Read the model definition and answer for the solid it produces. Units are mm, in the model's axes. Round coordinates to 2 decimals unless told otherwise and drop trailing zeros. Order: outer loops, then holes, each group sorted by start corner. A loop starts at its lowest first (then second) coordinate and runs counter-clockwise, first axis right, second up. Notation, with made-up numbers: (7, 72) - (40, 72) arc R29 cw to (40, 95) - close; hole circle Ø11 at (49.25, -22). An arc over 180 degrees is marked (long way). Put each result on its own line as item: value. Start each with the question number.
Q1. Section D-D on z = -3.75 is taken. Give the vertices of the cut face in (x, y).
Q2. Section B-B on x = -74 is taken. Give the vertices of the cut face in (y, z) (3 decimals), then the cut area to 3 significant figures.
Q3. Find the intervals of material crossed by line 1 along X through (y, z) = (0.75, -10.3); line 2 along X through (y, z) = (1.6, -11.75); line 3 along Y through (x, z) = (-8, -5), in increasing order. Write a range as from..to.
Q4. Section C-C on y = 1.35 is taken. Give the vertices of the cut face in (x, z).
Q5. This flat-tipped pin is pushed along its axis until it touches: pin 1 Ø1 at (x, z) = (-90, -5) entering from -Y. Where does it stop, or does it pass through?
Q6. Section A-A on z = -10.3 is taken. Give the vertices of the cut face in (x, y), then the cut area to 3 significant figures.
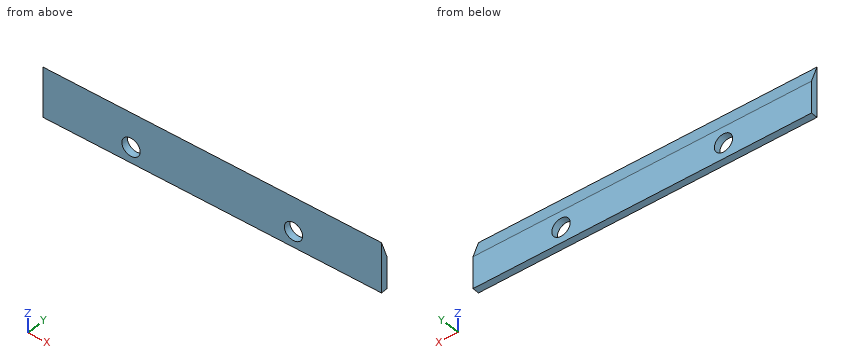
Autodesk Inventor part; units mm, degrees
ref_plane "Work Plane1" through (-50, 0, -15) normal (1, 0, 0) x (0, 0, -1)
ref_plane "YZ Plane" through (0, 0, 0) normal (1, 0, 0) x (0, 1, 0)
ref_plane "XZ Plane" through (0, 0, 0) normal (0, 1, 0) x (-1, 0, 0)
sketch "Sketch1" plane through (0, 0, 0) normal (0, 1, 0) x (-1, 0, 0)
  line L0 (0, 0) -> (100, 0)
  line L1 (100, 0) -> (100, -15)
  line L2 (100, -15) -> (0, -15)
  line L3 (0, -15) -> (0, 0)
  dimension "d0" = 100
  dimension "d1" = 15
extrude "Extrusion1" add sketch "Sketch1" along normal blind 2
sketch "Sketch2" plane through (0, 0, 0) normal (1, 0, 0) x (0, 0, -1)
  line L0 (0, 0) -> (0, 2)
  line L1 (0, 0) -> (5.495, 2)
  line L2 (5.495, 2) -> (5.495, 0)
  line L3 (5.495, 0) -> (0, 0)
  line L4 (0, 2) -> (15, 2)
  dimension "d4" = 20
extrude "Extrusion2" cut sketch "Sketch2" against normal through all contours L0 L4 L1
sketch "Sketch3" plane through (0, 2, 0) normal (0, 1, 0) x (1, 0, 0)
  line L0 (-100, 15) -> (-100, 5.495)
  point P0 (0, 0)
  point P1 (-74, 10.3)
  point P2 (-100, 10.2475)
  dimension "d14" = 26
  dimension "d15" = 4.7
hole "Hole1" at (-74, 2, -10.3) direction (0, -1, 0) diameter 5.4 depth 5.83
ref_plane "Work Plane1" through (-50, 0, -15) normal (1, 0, 0) x (0, 0, -1)
mirror "Mirror1" about plane through (-50, 0, -15) normal (1, 0, 0) of "Hole1"
properties part number "Blade"
Findings:
1. outline: (-100, 0) - (0, 0) - (0, 1.36) - (-100, 1.36) - close
2. outline: (0, -15) - (2, -15) - (2, -13) - (0, -13) - close; (0, -7.6) - (2, -7.6) - (2, -5.495) - (0, 0) - close
2. area: 13.7 mm2
3. line 1: -100..-76.7, -71.3..-28.7, -23.3..0
3. line 2: -100..-76.28, -71.72..-28.28, -23.72..0
3. line 3: 0..1.82
4. outline: (-100, -15) - (0, -15) - (0, -3.71) - (-100, -3.71) - close; hole circle Ø5.4 at (-74, -10.3); hole circle Ø5.4 at (-26, -10.3)
5. pin 1: y = 0
6. outline: (-100, 0) - (-76.7, 0) - (-76.7, 2) - (-100, 2) - close; (-71.3, 0) - (-28.7, 0) - (-28.7, 2) - (-71.3, 2) - close; (-23.3, 0) - (0, 0) - (0, 2) - (-23.3, 2) - close
6. area: 178 mm2
